Print and shaded views of the part. All mm, measured from the part's lowest x, y and z. A direction names the side the tool comes from. Round coordinates to 2 decimals unless told otherwise and drop trailing zeros. Loops run counter-clockwise (first coordinate to the right, second up) from the corner with the lowest first, then second, coordinate; pieces in that order, holes last. Notation, with made-up numbers: (74, -39) - (119, -39) arc R15 ccw to (119, -24) - close; hole circle Ø7 at (26.5, -10.75). An arc over 180 degrees is marked (long way). Answer as a JSON object with one key per item and string values.
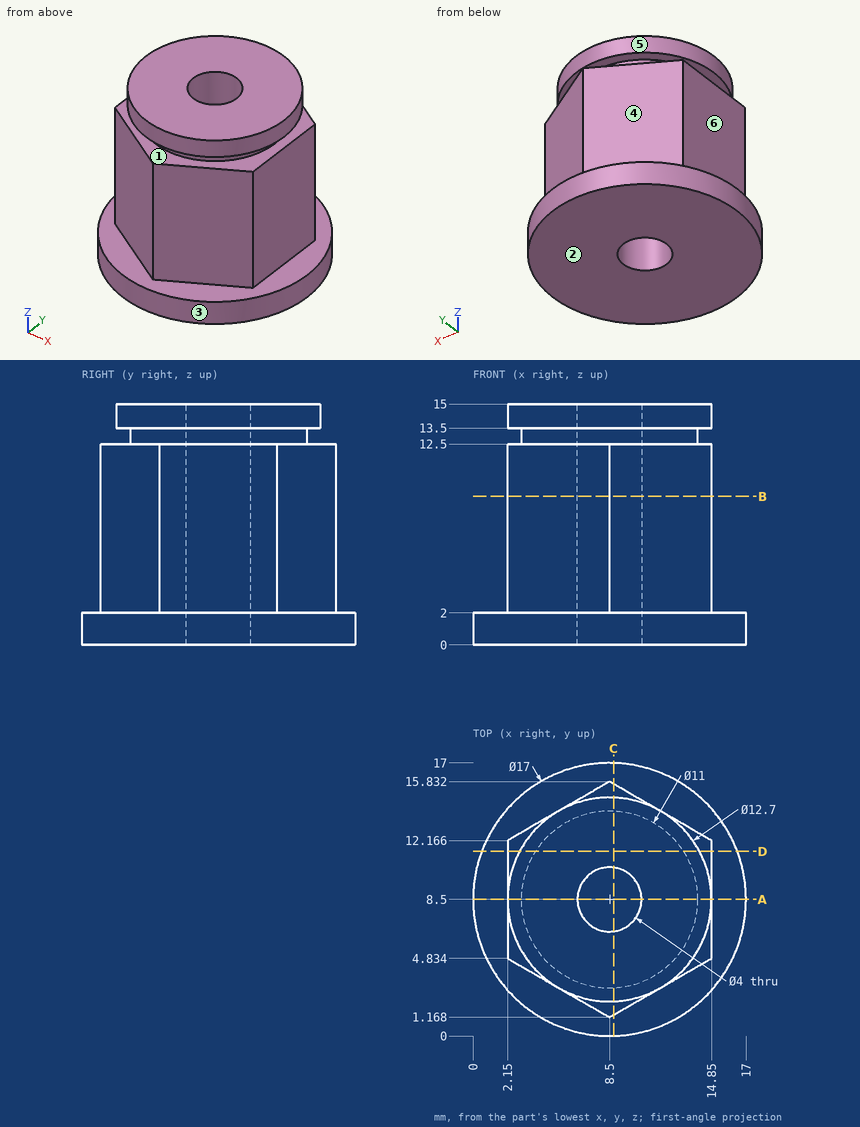
1) Slice it at A-A on y = 8.5. List the corners of the cut face in (x, z).
Values follow:
{"outline": "(0, 0) - (6.5, 0) - (6.5, 15) - (2.15, 15) - (2.15, 13.5) - (3, 13.5) - (3, 12.5) - (2.15, 12.5) - (2.15, 2) - (0, 2) - close; (10.5, 0) - (17, 0) - (17, 2) - (14.85, 2) - (14.85, 12.5) - (14, 12.5) - (14, 13.5) - (14.85, 13.5) - (14.85, 15) - (10.5, 15) - close"}
2) Probe probe 1 along Z at (x, y) = (3.75, 4.75); probe 2 along X at (y, z) = (11.5, 3.25); probe 3 along Y at (x, z) = (10, 6.25) (1 decimal). List the from-to ranges inside material, lowest first.
Values follow:
{"probe 1": "0 to 12.5, 13.5 to 15", "probe 2": "2.15 to 14.85", "probe 3": "2 to 7.2, 9.8 to 15"}
3) Tool access for the marked faces 4, 5 and 6: list every direction of +Z, -Z, +X, -X, +Y, -Y with a clear straight run to the whole face (end or side of a thin tool).
Values follow:
{"face 4": "+Z, -X, +Y", "face 5": "+Z", "face 6": "+Z, -X, +Y, -Y"}
4) Slice it at D-D on y = 11.5. List the corners of the cut face in (x, z).
Values follow:
{"outline": "(0.55, 0) - (16.45, 0) - (16.45, 2) - (14.85, 2) - (14.85, 12.5) - (13.11, 12.5) - (13.11, 13.5) - (14.1, 13.5) - (14.1, 15) - (2.9, 15) - (2.9, 13.5) - (3.89, 13.5) - (3.89, 12.5) - (2.15, 12.5) - (2.15, 2) - (0.55, 2) - close"}
5) Slice it at B-B on z = 9.25. List the corners of the cut face in (x, y), then the cut area to 3 significant figures.
Values follow:
{"outline": "(2.15, 4.83) - (8.5, 1.17) - (14.85, 4.83) - (14.85, 12.17) - (8.5, 15.83) - (2.15, 12.17) - close; hole circle Ø4 at (8.5, 8.5)", "area": "127 mm²"}
6) Drop flat-ended pins along their axis: P1, Ø5, axis at y = 6, z = 8.5, coming from the -X side; P2, Ø2, axis at y = 9, z = 8.5, coming from the +X side; P3, Ø2, axis at x = 10.5, z = 2, coming from the +Y side. Give the stop position or say it passes through.
Values follow:
{"P1": "x = 2.15", "P2": "x = 14.85", "P3": "y = 16.94"}
7) Two-plate mould, pull along Z, no slides. Class the marked faces 1, 2 and 3: pulls with the +Z half, pulls with the -Z half, needs draft (parallel to the pull), parting line crosses it, or undercut.
Values follow:
{"face 1": "undercut", "face 2": "pulls with the -Z half", "face 3": "needs draft"}
8) Slice it at C-C on x = 8.75. List the corners of the cut face in (y, z) (1 decimal).
Values follow:
{"outline": "(0, 0) - (6.5, 0) - (6.5, 15) - (2.2, 15) - (2.2, 13.5) - (3, 13.5) - (3, 12.5) - (1.3, 12.5) - (1.3, 2) - (0, 2) - close; (10.5, 0) - (17, 0) - (17, 2) - (15.7, 2) - (15.7, 12.5) - (14, 12.5) - (14, 13.5) - (14.8, 13.5) - (14.8, 15) - (10.5, 15) - close"}
